from build123d import *

# Parameters (mm, degrees)
SKETCH1_W           = 190.5
SKETCH1_H           = 175
BOSS_EXTRUDE1_DEPTH = 40
SHELL1_T            = -15
SKETCH2_W           = 175
SKETCH2_H           = 4.9
BOSS_EXTRUDE2_DEPTH = 5
SKETCH3_W           = 5
SKETCH3_H           = 5
CUT_EXTRUDE1_DEPTH  = 175
SKETCH4_W           = 7.5
SKETCH4_H           = 145
CUT_EXTRUDE2_DEPTH  = 25
CUT_EXTRUDE3_START  = -190.5
SKETCH5_R           = 2.65
SKETCH5_R_2         = 2.15
CUT_EXTRUDE3_DEPTH  = 190.5
SKETCH6_W           = 168
SKETCH6_H           = 145
CUT_EXTRUDE4_DEPTH  = 7.5
CUT_EXTRUDE5_REACH  = 140.947
SKETCH7_W           = 9
SKETCH7_H           = 144.996152815
BOSS_EXTRUDE3_START = -7.5
SKETCH9_W           = 190.5
SKETCH9_H           = 5
BOSS_EXTRUDE3_DEPTH = 2.45
SKETCH11_R          = 1.65
CUT_EXTRUDE7_DEPTH  = 4.9
SKETCH12_W          = 35
SKETCH12_H          = 25
CUT_EXTRUDE8_DEPTH  = 213.19154083
CUT_EXTRUDE9_REACH  = 214.192
SKETCH13_W          = 15
SKETCH13_H          = 25


with BuildPart() as part:
    # Sketch1 → Boss-Extrude1 (new body)
    with BuildSketch(Plane(origin=(0, 0, 0), x_dir=(1, 0, 0), z_dir=(0, 1, 0))):
        Rectangle(SKETCH1_W, SKETCH1_H)
    extrude(amount=BOSS_EXTRUDE1_DEPTH)

    # Shell1
    shell1_openings = [part.faces().sort_by_distance(p)[0] for p in [
        (0, 40, 0),
    ]]
    offset(amount=SHELL1_T, openings=shell1_openings, kind=Kind.INTERSECTION)

    # Sketch2 → Boss-Extrude2 (add)
    with BuildSketch(Plane(origin=(95.25, 0, 0), x_dir=(0, 0, -1), z_dir=(1, 0, 0))):
        with Locations((0, 20)):
            Rectangle(SKETCH2_W, SKETCH2_H)
    extrude(amount=BOSS_EXTRUDE2_DEPTH)

    # Sketch3 → Cut-Extrude1 (cut)
    with BuildSketch(Plane.XY.offset(87.5)):
        with Locations((-92.75, 20)):
            Rectangle(SKETCH3_W, SKETCH3_H)
    extrude(amount=-CUT_EXTRUDE1_DEPTH, mode=Mode.SUBTRACT)

    # Sketch4 → Cut-Extrude2 (cut)
    with BuildSketch(Plane(origin=(0, 40, 0), x_dir=(1, 0, 0), z_dir=(0, 1, 0))):
        with Locations((-84, 0)):
            Rectangle(SKETCH4_W, SKETCH4_H)
    extrude(amount=-CUT_EXTRUDE2_DEPTH, mode=Mode.SUBTRACT)

    # Sketch5 → Cut-Extrude3 (cut)
    with BuildSketch(Plane.ZY.offset(95.25).offset(CUT_EXTRUDE3_START)):
        with Locations((0, 30)):
            Circle(SKETCH5_R)
        with Locations((-30, 30)):
            Circle(SKETCH5_R_2)
        with Locations((50, 30)):
            Circle(SKETCH5_R_2)
        with Locations((-30, 13.5)):
            Circle(SKETCH5_R_2)
        with Locations((0, 13.5)):
            Circle(SKETCH5_R)
        with Locations((50, 13.5)):
            Circle(SKETCH5_R_2)
    cut_extrude3 = extrude(amount=CUT_EXTRUDE3_DEPTH, mode=Mode.SUBTRACT)

    # Sketch6 → Cut-Extrude4 (cut)
    with BuildSketch(Plane(origin=(0, 15, 0), x_dir=(1, 0, 0), z_dir=(0, 1, 0))):
        with Locations((-3.75, 0)):
            Rectangle(SKETCH6_W, SKETCH6_H)
    extrude(amount=-CUT_EXTRUDE4_DEPTH, mode=Mode.SUBTRACT)

    # Mirror1: Cut-Extrude3 across plane
    add(cut_extrude3.mirror(Plane(origin=(0, 0, 0), x_dir=(0, 0, 1), z_dir=(1, 0, 0))), mode=Mode.SUBTRACT)

    # Cut-Extrude5: up to this face of the body (flat: up to its plane)
    cut_extrude5_end = Plane(part.part.faces().sort_by_distance((-3.75, 7.5, 0))[0])
    # Sketch7 → Cut-Extrude5 (cut, up to the picked face)
    with BuildSketch(Plane(origin=(0, 40, 0), x_dir=(1, 0, 0), z_dir=(0, 1, 0)), mode=Mode.PRIVATE) as cut_extrude5_sk1:
        with Locations((84.75, 0.001923592)):
            Rectangle(SKETCH7_W, SKETCH7_H)
    cut_extrude5_tool1 = split(extrude(cut_extrude5_sk1.sketch, amount=-CUT_EXTRUDE5_REACH, mode=Mode.PRIVATE), bisect_by=cut_extrude5_end, keep=Keep.BOTH, mode=Mode.PRIVATE)
    add(cut_extrude5_tool1.solids().sort_by(Axis((84.75, 40, -0.001924), (0, -1, 0)))[0], mode=Mode.SUBTRACT)

    # Sketch9 → Boss-Extrude3 (add, symmetric)
    with BuildSketch(Plane.XY.offset(87.5).offset(BOSS_EXTRUDE3_START)):
        with Locations((0, 42.5)):
            Rectangle(SKETCH9_W, SKETCH9_H)
    boss_extrude3 = extrude(amount=BOSS_EXTRUDE3_DEPTH, both=True)

    # Sketch11 → Cut-Extrude7 (cut)
    with BuildSketch(Plane(origin=(0, 0, 77.55), x_dir=(-1, 0, 0), z_dir=(0, 0, -1))):
        with Locations((-80, 42.5)):
            Circle(SKETCH11_R)
        with Locations((80, 42.5)):
            Circle(SKETCH11_R)
    cut_extrude7 = extrude(amount=-CUT_EXTRUDE7_DEPTH, mode=Mode.SUBTRACT)

    # Mirror2: Boss-Extrude3, Cut-Extrude7 across plane
    add(boss_extrude3.mirror(Plane.XY))
    add(cut_extrude7.mirror(Plane.XY), mode=Mode.SUBTRACT)

    # Sketch12 → Cut-Extrude8 (cut, through all)
    with BuildSketch(Plane(origin=(-87.75, 0, 0), x_dir=(0, 0, -1), z_dir=(1, 0, 0))):
        with Locations((-25, 20)):
            Rectangle(SKETCH12_W, SKETCH12_H)
    extrude(amount=CUT_EXTRUDE8_DEPTH, mode=Mode.SUBTRACT)

    # Cut-Extrude9: up to this face of the body (flat: up to its plane)
    cut_extrude9_end = Plane(part.part.faces().sort_by_distance((-95.25, 8.669388557, -0.096447103))[0])
    # Sketch13 → Cut-Extrude9 (cut, up to the picked face)
    with BuildSketch(Plane(origin=(-87.75, 0, 0), x_dir=(0, 0, -1), z_dir=(1, 0, 0)), mode=Mode.PRIVATE) as cut_extrude9_sk1:
        with Locations((-62.5, 20)):
            Rectangle(SKETCH13_W, SKETCH13_H)
    cut_extrude9_tool1 = split(extrude(cut_extrude9_sk1.sketch, amount=-CUT_EXTRUDE9_REACH, mode=Mode.PRIVATE), bisect_by=cut_extrude9_end, keep=Keep.BOTH, mode=Mode.PRIVATE)
    add(cut_extrude9_tool1.solids().sort_by(Axis((-87.75, 20, 62.5), (-1, 0, 0)))[0], mode=Mode.SUBTRACT)


solid = part.part
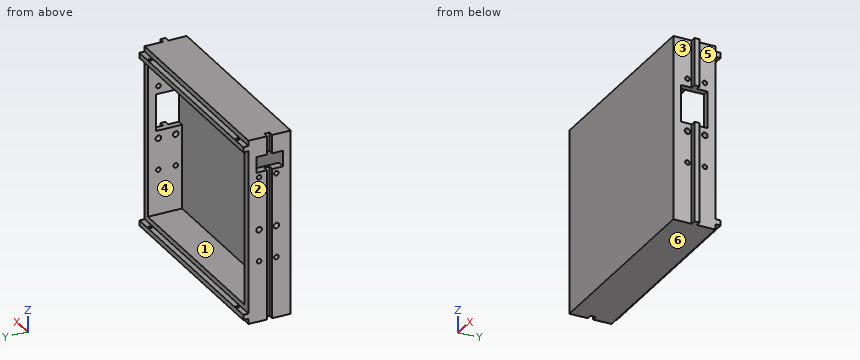
For this review, take the finished solid that the model builds, in its own axes (mm). Face numbers are marked on the shaded views. A direction names the side the tool comes from. Round coordinates to 2 decimals unless told otherwise and drop trailing zeros. Loops run counter-clockwise (first coordinate to the right, second up) from the corner with the lowest first, then second, coordinate; pieces in that order, holes last. Notation, with made-up numbers: (33, 67) - (54, 67) arc R17 ccw to (54, 72) - close; hole circle Ø6 at (76.25, 61.5). An arc over 180 degrees is marked (long way). Put each result on its own line as item: value. Start each with the question number.
1. Insertion check: P1, Ø12, axis at y = 7.5, z = 70, coming from the +X side; P2, Ø3.5, axis at x = 95.5, y = 14.5, coming from the +Z side; P3, Ø2, axis at x = 72.5, z = 25.5, coming from the +Y side; P4, Ø2.5, axis at x = -5.5, z = 86, coming from the +Y side. Each pin has a flat end and moves straight along its axis. Give the tip position at first contact, or say it passes through.
2. Consider section A-A on z = 66.5. State the section outline as (x, y) points.
3. Consider section D-D on z = 0. State how many separate pieces and enclosed holes the cut face has, plus the area to 3 significant figures.
4. For probe 1 along Y at (x, z) = (-91.5, 0); probe 2 along Z at (x, y) = (93.25, 13.5); probe 3 along Y at (x, z) = (91.65, 50), list the stretches that pass through material, from the lowest coordinate up. Write a range as [from, to].
5. For the marked faces 5 and 6, list the 3-axis set-ups (+Z, -Z, +X, -X, +Y, -Y) from which the entire face can be reached by the end or side of a thin tool; tool diameter is ignored.
6. Consider section C-C on x = -36. State the section outline as (y, z) points, plus the area to 3 significant figures.
7. Mouldability with a two-part tool opening along X and no side actions: class the marked faces 1, 2, 3 and 4 as +X half, -X half, draft (parallel to the pull), parting line (faces both ways), or undercut.
Result sheet:
1. P1: x = 95.25
1. P2: z = 87.5
1. P3: y = 7.5
1. P4: y = 40
2. outline: (-95.25, 0) - (95.25, 0) - (95.25, 17.55) - (100.25, 17.55) - (100.25, 22.45) - (95.25, 22.45) - (95.25, 40) - (89.25, 40) - (89.25, 7.5) - (-95.25, 7.5) - close; (-95.25, 32.5) - (-87.75, 32.5) - (-87.75, 40) - (-95.25, 40) - close
3. separate pieces: 5
3. enclosed holes: 0
3. area: 1,720 mm^2
4. probe 1: [0, 10.85], [16.15, 17.5], [22.5, 27.35], [32.65, 40]
4. probe 2: [-87.5, -32.15], [-27.85, -2.65], [2.65, 7.5], [42.5, 47.85], [52.15, 87.5]
4. probe 3: [0, 11.35], [15.65, 27.85], [32.15, 40]
5. face 5: +Z, -Z, +X, +Y
5. face 6: -Z, +X, -X, +Y, -Y
6. outline: (0, -87.5) - (40, -87.5) - (40, -82.45) - (45, -82.45) - (45, -77.55) - (40, -77.55) - (40, -72.5) - (7.5, -72.5) - (7.5, 72.5) - (40, 72.5) - (40, 77.55) - (45, 77.55) - (45, 82.45) - (40, 82.45) - (40, 87.5) - (0, 87.5) - close
6. area: 2,340 mm^2
7. face 1: undercut
7. face 2: -X half
7. face 3: +X half
7. face 4: undercut
